from build123d import *

# Parameters (mm, degrees)
ESQUISSE1_R        = 2.5
BOSS_EXTRU_1_DEPTH = 5
CONG_1_R           = 1
CONG_2_R           = 0.25


with BuildPart() as part:
    # Esquisse1 → Boss.-Extru.1 (new body)
    with BuildSketch(Plane.XY):
        with BuildLine():
            Line((-3.799671038, 1.25), (-17.299671038, 1.25))
            Line((-17.299671038, 1.25), (-25.299671038, 4))
            Line((-25.299671038, 4), (-45.299671038, 0))
            Line((-45.299671038, 0), (-25.299671038, -4))
            Line((-25.299671038, -4), (-17.170505914, -1.25))
            Line((-17.170505914, -1.25), (-3.799671038, -1.25))
            ThreePointArc((-3.799671038, -1.25), (4, 0), (-3.799671038, 1.25))
        make_face()
        Circle(ESQUISSE1_R, mode=Mode.SUBTRACT)
    extrude(amount=BOSS_EXTRU_1_DEPTH)

    # Congé1
    cong_1_edges = [part.edges().sort_by_distance(p)[0] for p in [
        (-25.299671038, 4, 2.5),
        (-17.299671038, 1.25, 2.5),
        (-3.799671038, 1.25, 2.5),
        (-3.799671038, -1.25, 2.5),
        (-17.170505914, -1.25, 2.5),
        (-25.299671038, -4, 2.5),
    ]]
    fillet(cong_1_edges, radius=CONG_1_R)

    # Congé2
    cong_2_edges = [part.edges().sort_by_distance(p)[0] for p in [
        (-45.299671038, 0, 2.5),
    ]]
    fillet(cong_2_edges, radius=CONG_2_R)


solid = part.part
For this review, take the finished solid that the model builds, in its own axes (mm). A direction names the side the tool comes from. Coordinates: 2 decimals unless noted, no trailing zeros. Order: outer loops, then holes, each group sorted by start corner. A loop starts at its lowest first (then second) coordinate and runs counter-clockwise, first axis right, second up. Notation, with made-up numbers: (35, 31.25) - (82, 31.25) arc R24 cw to (82, 51.25) - close; hole circle Ø1 at (69, 88). An arc over 180 degrees is marked (long way). Use one line per item in the form item = value.
Q1. For P1, Ø3, axis at x = 0, y = 0, coming from the +Z side, flat-tipped, find the tip position at first contact; note if it passes through.
Checked values:
P1 = through
Q2. Consider section D-D (x = -28). Give the boundary of the cut face in (y, z), then the cut area to 3 significant figures.
Checked values:
outline = (-3.46, 0) - (3.46, 0) - (3.46, 5) - (-3.46, 5) - close
area = 34.6 mm2
Q3. For faces 4 (the cylindrical face through (-3.947, 1.395, 2.535)), 5 (the cylindrical face through (-3.934, -1.403, 2.535)), 6 (the cylindrical face through (4, 0, 2)), list the 3-axis set-ups (+Z, -Z, +X, -X, +Y, -Y) from which the entire face can be reached by the end or side of a thin tool; tool diameter is ignored.
Checked values:
face_4 = +Z, -Z, +Y
face_5 = +Z, -Z, -Y
face_6 = +Z, -Z
Q4. Consider section B-B (z = 3.8). Give the boundary of the cut face in (x, y).
Checked values:
outline = (-44.07, -0.25) - (-25.56, -3.95) arc R1 ccw to (-25.05, -3.91) - (-17.33, -1.3) arc R1 cw to (-17.01, -1.25) - (-4.47, -1.25) arc R1 cw to (-3.57, -1.8) arc R4 ccw (long way) to (-3.57, 1.8) arc R1 cw to (-4.47, 1.25) - (-17.13, 1.25) arc R1 cw to (-17.46, 1.3) - (-25.04, 3.91) arc R1 ccw to (-25.56, 3.95) - (-44.07, 0.25) arc R0.25 ccw to start; hole circle Ø5 at (0, 0)
Q5. Consider section A-A (x = 0). Give the boundary of the cut face in (y, z).
Checked values:
outline = (-4, 0) - (-2.5, 0) - (-2.5, 5) - (-4, 5) - close; (2.5, 0) - (4, 0) - (4, 5) - (2.5, 5) - close
Q6. Consider section C-C (y = -0.75). Give the boundary of the cut face in (x, z).
Checked values:
outline = (-41.55, 0) - (-2.38, 0) - (-2.38, 5) - (-41.55, 5) - close; (2.38, 0) - (3.93, 0) - (3.93, 5) - (2.38, 5) - close
Q7. For probe 1 along Y at (x, z) = (0, 2.2); probe 2 along Y at (x, z) = (-12, 1.8); probe 3 along Y at (x, z) = (-25.5, 0.85), list the stretches that pass through material, from the lowest coordinate up. Write a range as from..to.
Checked values:
probe_1 = -4..-2.5, 2.5..4
probe_2 = -1.25..1.25
probe_3 = -3.96..3.96
Q8. Draft analysis for pull direction Y (two halves, no side actions). For faces 1 (the flat face through (-11, -1.25, 2)), 2 (the flat face through (-21.2, 2.59, 2.46)), 3 (the cylindrical face through (-0.54, -2.44, 2.46)), state which applies: +Y half, -Y half, draft (parallel to the pull), parting line (faces both ways), or undercut.
Checked values:
face_1 = -Y half
face_2 = +Y half
face_3 = undercut
